The model under review builds one solid part; all positions refer to its coordinate system, in mm. Face numbers are marked on the shaded views. A direction names the side the tool comes from. Coordinates: 2 decimals unless noted, no trailing zeros. Order: outer loops, then holes, each group sorted by start corner. A loop starts at its lowest first (then second) coordinate and runs counter-clockwise, first axis right, second up. Notation, with made-up numbers: (-10, -0.5) -> (21, -0.5) arc R28 ccw to (21, 34.5) -> close; hole circle Ø5 at (-36, 73). An arc over 180 degrees is marked (long way). Use one line per item in the form item = value.
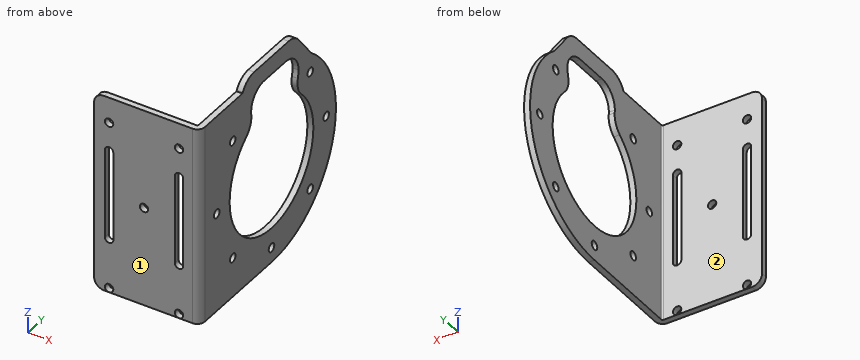
from build123d import *

# Parameters (mm, degrees)
SKETCH_1_R                       = 2.15
SM_BASE_FLANGE_1_DEPTH           = 3
SM_EDGE_FLANGE_1_STRIP_W         = 13.4732
SM_EDGE_FLANGE_1_STRIP_H         = 3
SM_EDGE_FLANGE_1_STRIP_CUT_DEPTH = 100
SM_EDGE_FLANGE_1_DEPTH           = 100
SKETCH_9_R                       = 2.1
CUT_EXTRUDE_1_DEPTH              = 10
FILLET_1_R                       = 5
SKETCH_10_R                      = 2.1
CUT_EXTRUDE_2_DEPTH              = 10


# Sheet-metal steps are written as plain solids
with BuildPart() as part:
    # Sketch 1 → 基体-法兰1 (new body)
    with BuildSketch(Plane(origin=(0, 0, 0), x_dir=(0, 0, -1), z_dir=(1, 0, 0))):
        with BuildLine():
            Line((-50, -22.510788707), (-50, -55.5))
            Line((-50, -55.5), (50, -55.5))
            Line((50, -55.5), (50, 0))
            ThreePointArc((50, 0), (16.339860062, 47.254724348), (-39.320358927, 30.885423324))
            Line((-39.320358927, 30.885423324), (-51.83191014, 21.160585638))
            ThreePointArc((-51.83191014, 21.160585638), (-54.677464079, 17.660055501), (-55.695008503, 13.265116159))
            Line((-55.695008503, 13.265116159), (-55.695008503, -13.471087591))
            ThreePointArc((-55.695008503, -13.471087591), (-54.312022765, -18.545244191), (-50.545595463, -22.215903549))
            ThreePointArc((-50.545595463, -22.215903549), (-50.273602999, -22.364836031), (-50, -22.510788707))
        make_face()
        with Locations((0, 42.5)):
            Circle(SKETCH_1_R, mode=Mode.SUBTRACT)
        with Locations((30.0520382, 30.0520382)):
            Circle(SKETCH_1_R, mode=Mode.SUBTRACT)
        with Locations((42.5, 0)):
            Circle(SKETCH_1_R, mode=Mode.SUBTRACT)
        with Locations((30.0520382, -30.0520382)):
            Circle(SKETCH_1_R, mode=Mode.SUBTRACT)
        with Locations((0, -42.5)):
            Circle(SKETCH_1_R, mode=Mode.SUBTRACT)
        with Locations((-30.0520382, -30.0520382)):
            Circle(SKETCH_1_R, mode=Mode.SUBTRACT)
        with Locations((-30.0520382, 30.0520382)):
            Circle(SKETCH_1_R, mode=Mode.SUBTRACT)
        with BuildLine():
            Line((-46.595603285, 10.997841176), (-46.595603285, -5.777394466))
            ThreePointArc((-46.595603285, -5.777394466), (-43.590659136, -12.923665777), (-36.381764555, -15.775107854))
            ThreePointArc((-36.381764555, -15.775107854), (-35.646197226, -15.744635296), (-34.912439019, -15.684745692))
            ThreePointArc((-34.912439019, -15.684745692), (-29.904748182, -16.465924493), (-25.923223086, -19.601951556))
            ThreePointArc((-25.923223086, -19.601951556), (32.418442092, -2.301002457), (-22.894661052, 23.066956784))
            ThreePointArc((-22.894661052, 23.066956784), (-27.279217704, 20.524739091), (-32.347042381, 20.45870218))
            ThreePointArc((-32.347042381, 20.45870218), (-34.349504558, 20.839101356), (-36.381764555, 20.995554565))
            ThreePointArc((-36.381764555, 20.995554565), (-43.590659136, 18.144112487), (-46.595603285, 10.997841176))
        make_face(mode=Mode.SUBTRACT)
    extrude(amount=-SM_BASE_FLANGE_1_DEPTH)

    # 边线-法兰1 strip (across the edge) → 边线-法兰1 strip cut (cut)
    with BuildSketch(Plane(origin=(-3, -55.5, -50), x_dir=(0, 1, 0), z_dir=(0, 0, 1))):
        with Locations((-3, -1.5)):
            Rectangle(SM_EDGE_FLANGE_1_STRIP_W, SM_EDGE_FLANGE_1_STRIP_H)
    extrude(amount=SM_EDGE_FLANGE_1_STRIP_CUT_DEPTH, mode=Mode.SUBTRACT)

    # 边线-法兰1 section (across the edge) → 边线-法兰1 (add)
    with BuildSketch(Plane(origin=(-3, -55.5, -50), x_dir=(0, 1, 0), z_dir=(0, 0, 1))):
        with BuildLine():
            Line((0, 0.7366), (0, 50))
            Line((0, 50), (3, 50))
            Line((3, 50), (3, 0.7366))
            ThreePointArc((3, 0.7366), (3.215745145, 0.215745145), (3.7366, 0))
            Line((3.7366, 0), (3.7366, -3))
            ThreePointArc((3.7366, -3), (1.094424801, -1.905575199), (0, 0.7366))
        make_face()
    extrude(amount=SM_EDGE_FLANGE_1_DEPTH)

    # 草图9 → 切除-拉伸1 (cut)
    with BuildSketch(Plane(origin=(0, -52.5, 0), x_dir=(1, 0, 0), z_dir=(0, 1, 0))):
        with Locations(Location((-45.5, 47.839820537, 0), (0, 0, 180))):
            Circle(SKETCH_9_R)
        with Locations(Location((-10.5, 47.839820537, 0), (0, 0, 180))):
            Circle(SKETCH_9_R)
        with Locations(Location((-45.5, -37.160179463, 0), (0, 0, 180))):
            Circle(SKETCH_9_R)
        with Locations(Location((-10.5, -37.160179463, 0), (0, 0, 180))):
            Circle(SKETCH_9_R)
    extrude(amount=-CUT_EXTRUDE_1_DEPTH, mode=Mode.SUBTRACT)

    # 圆角1
    fillet_1_edges = [part.edges().sort_by_distance(p)[0] for p in [
        (-53, -54, -50),
        (-53, -54, 50),
    ]]
    fillet(fillet_1_edges, radius=FILLET_1_R)

    # 草图10 → 切除-拉伸2 (cut)
    with BuildSketch(Plane(origin=(0, -52.5, 0), x_dir=(1, 0, 0), z_dir=(0, 1, 0))):
        with Locations(Location((-28, 0, 0), (0, 0, 180))):
            Circle(SKETCH_10_R)
        with BuildLine():
            Line((-43.4, 22.5), (-43.4, -22.5))
            ThreePointArc((-43.4, -22.5), (-45.5, -24.6), (-47.6, -22.5))
            Line((-47.6, -22.5), (-47.6, 22.5))
            ThreePointArc((-47.6, 22.5), (-45.5, 24.6), (-43.4, 22.5))
        make_face()
        with BuildLine():
            Line((-8.4, 22.5), (-8.4, -22.5))
            ThreePointArc((-8.4, -22.5), (-10.5, -24.6), (-12.6, -22.5))
            Line((-12.6, -22.5), (-12.6, 22.5))
            ThreePointArc((-12.6, 22.5), (-10.5, 24.6), (-8.4, 22.5))
        make_face()
    extrude(amount=-CUT_EXTRUDE_2_DEPTH, mode=Mode.SUBTRACT)


solid = part.part
Item 1: Tool access review of the marked faces 1 and 2: name each direction out of +Z, -Z, +X, -X, +Y, -Y from which nothing blocks a thin tool from reaching the whole face with its end or side.
Results found:
face_1 = +Z, -Z, +X, -X, -Y
face_2 = +Z, -Z, -X, +Y
Item 2: To check wall thickness, follow L1, parallel to Y at x = -0.9, z = 0; L2, parallel to Y at x = -22, z = -7; L3, parallel to Y at x = -2, z = 0. State the ranges of each line that lie inside material, in increasing order. Write a range as from..to.
Results found:
L1 = -54.2..-44.65, -40.35..-32.5, 32.5..40.35, 44.65..50
L2 = -55.5..-52.5
L3 = -55.07..-44.65, -40.35..-32.5, 32.5..40.35, 44.65..50
Item 3: We need section A-A (y = -42.5). Write out the cut boundary in (x, z).
Results found:
outline = (-3, -50) -> (0, -50) -> (0, -2.15) -> (-3, -2.15) -> close; (-3, 2.15) -> (0, 2.15) -> (0, 50) -> (-3, 50) -> close
Item 4: We need section B-B (x = -45.5). Write out the cut boundary in (y, z), plus the area to 3 significant figures.
Results found:
outline = (-55.5, -50) -> (-52.5, -50) -> (-52.5, -49.94) -> (-55.5, -49.94) -> close; (-55.5, -45.74) -> (-52.5, -45.74) -> (-52.5, -24.6) -> (-55.5, -24.6) -> close; (-55.5, 24.6) -> (-52.5, 24.6) -> (-52.5, 35.06) -> (-55.5, 35.06) -> close; (-55.5, 39.26) -> (-52.5, 39.26) -> (-52.5, 50) -> (-55.5, 50) -> close
area = 127 mm²
Item 5: We need section D-D (z = 16). Write out the cut boundary in (x, y).
Results found:
outline = (-53, -55.5) -> (-47.6, -55.5) -> (-47.6, -52.5) -> (-53, -52.5) -> close; (-43.4, -55.5) -> (-12.6, -55.5) -> (-12.6, -52.5) -> (-43.4, -52.5) -> close; (-8.4, -55.5) -> (-3.74, -55.5) arc R3.74 ccw to (0, -51.76) -> (0, -28.29) -> (-3, -28.29) -> (-3, -51.76) arc R0.74 cw to (-3.74, -52.5) -> (-8.4, -52.5) -> close; (-3, 28.29) -> (0, 28.29) -> (0, 47.37) -> (-3, 47.37) -> close
Item 6: We need section C-C (z = -26). Write out the cut boundary in (x, y), plus the area to 3 significant figures.
Results found:
outline = (-53, -55.5) -> (-3.74, -55.5) arc R3.74 ccw to (0, -51.76) -> (0, -19.5) -> (-3, -19.5) -> (-3, -51.76) arc R0.74 cw to (-3.74, -52.5) -> (-53, -52.5) -> close; (-3, 19.5) -> (0, 19.5) -> (0, 42.71) -> (-3, 42.71) -> close
area = 325 mm²
Item 7: Clearance check with flat-ended pins moving along their axes: pin 1 (2.5 mm diameter, centred on x = -45.5, z = 37.16, fed in from -Y); pin 2 (5.5 mm diameter, centred on y = -30.05, z = 30.05, fed in from -X); pin 3 (2.5 mm diameter, centred on y = -53.5, z = -5, fed in from +X); pin 4 (2 mm diameter, centred on x = -20.5, z = 36.5, fed in from +Y). State where each tip first meets the part, or that it passes through.
Results found:
pin_1 = through
pin_2 = -3
pin_3 = -0.03
pin_4 = -52.5
